Design review of the part built by this model. Coordinates are the model's own, in mm. A direction names the side the tool comes from. Coordinates: 2 decimals unless noted, no trailing zeros. Order: outer loops, then holes, each group sorted by start corner. A loop starts at its lowest first (then second) coordinate and runs counter-clockwise, first axis right, second up. Notation, with made-up numbers: (3.25, -21.75) - (26.25, -21.75) arc R10 ccw to (26.25, -9.75) - close; hole circle Ø4 at (-30.75, 59). An arc over 180 degrees is marked (long way). Write each question's results on one line, items separated by ' | '. Start each with the question number.
```python
from build123d import *

# Parameters (mm, degrees)
ESQUISSE1_R        = 6.5
ESQUISSE1_R_2      = 2.75
BOSS_EXTRU_1_DEPTH = 3.5
ESQUISSE2_R        = 6.5
BOSS_EXTRU_2_DEPTH = 2
ESQUISSE3_R        = 2.5
BOSS_EXTRU_3_DEPTH = 3
CHANFREIN1_SIZE    = 0.5


with BuildPart() as part:
    # Esquisse1 → Boss.-Extru.1 (new body)
    with BuildSketch(Plane.XY):
        Circle(ESQUISSE1_R)
        Circle(ESQUISSE1_R_2, mode=Mode.SUBTRACT)
    extrude(amount=BOSS_EXTRU_1_DEPTH)

    # Esquisse2 → Boss.-Extru.2 (add)
    with BuildSketch(Plane.XY.offset(3.5)):
        Circle(ESQUISSE2_R)
    extrude(amount=BOSS_EXTRU_2_DEPTH)

    # Esquisse3 → Boss.-Extru.3 (add)
    with BuildSketch(Plane.XY.offset(5.5)):
        Circle(ESQUISSE3_R)
    extrude(amount=BOSS_EXTRU_3_DEPTH)

    # Chanfrein1
    chanfrein1_edges = [part.edges().sort_by_distance(p)[0] for p in [
        (-2.5, 0, 8.5),
    ]]
    chamfer(chanfrein1_edges, length=CHANFREIN1_SIZE)


solid = part.part
```
(1) Take a section at C-C (z = 1.75). State the section outline as (x, y) points, plus the area to 3 significant figures.
(2) Take a section at D-D (z = 5.75). State the section outline as (x, y) points, plus the area to 3 significant figures.
(3) Take a section at A-A (x = 0). State the section outline as (y, z) points, plus the area to 3 significant figures.
(4) Mouldability with a two-part tool opening along X and no side actions: class faces 1 (the face through (3, 0, 0)), 2 (the face through (-0.596, -2.685, 1.726)), 3 (the face through (-0.54, -2.44, 6.73)), 4 (the face through (0, 0, 3.5)) as +X half, -X half, draft (parallel to the pull), parting line (faces both ways), or undercut.
(5) Tool access review of faces 5 (the face through (0, 0, 8.5)), 6 (the face through (3, 0, 5.5)): name each direction out of +Z, -Z, +X, -X, +Y, -Y from which nothing blocks a thin tool from reaching the whole face with its end or side.
(6) Clearance check with flat-ended pins moving along their axes: pin 1 (1 mm diameter, centred on x = 4.5, z = 1.5, fed in from -Y); pin 2 (1.5 mm diameter, centred on x = 0, y = -4.5, fed in from +Z); pin 3 (1 mm diameter, centred on x = -5, z = 2, fed in from -Y). State where each tip first meets the part, or that it passes through.
(7) To check wall thickness, follow line 1 along Y through (x, z) = (0, 1.6); line 2 along Z through (x, y) = (-3.75, 0.5); line 3 along X through (y, z) = (-2, 2.25). State the ranges of each line that lie inside material, in increasing order. Write a range as [from, to].
Worked out:
1) outline: circle Ø13 at (0, 0); hole circle Ø5.5 at (0, 0) | area: 109 mm^2
2) outline: circle Ø5 at (0, 0) | area: 19.6 mm^2
3) outline: (-6.5, 0) - (-2.75, 0) - (-2.75, 3.5) - (2.75, 3.5) - (2.75, 0) - (6.5, 0) - (6.5, 5.5) - (2.5, 5.5) - (2.5, 8) - (2, 8.5) - (-2, 8.5) - (-2.5, 8) - (-2.5, 5.5) - (-6.5, 5.5) - close | area: 67.0 mm^2
4) face 1: draft | face 2: undercut | face 3: parting line | face 4: undercut
5) face 5: +Z, +X, -X, +Y, -Y | face 6: +Z
6) pin 1: y = -5.12 | pin 2: z = 5.5 | pin 3: y = -4.69
7) line 1: [-6.5, -2.75], [2.75, 6.5] | line 2: [0, 5.5] | line 3: [-6.18, -1.89], [1.89, 6.18]
